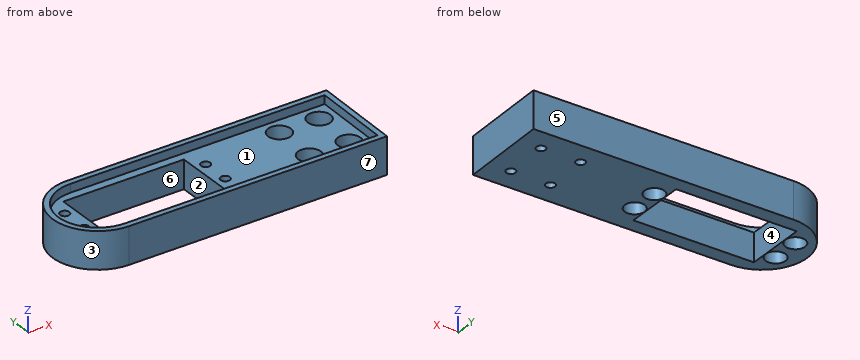
Autodesk Inventor part; units mm, degrees
ref_plane "YZ Plane" through (0, 0, 0) normal (1, 0, 0) x (0, 1, 0)
ref_plane "XZ Plane" through (0, 0, 0) normal (0, 1, 0) x (-1, 0, 0)
ref_plane "XY Plane" through (0, 0, 0) normal (0, 0, 1) x (1, 0, 0)
sketch "Szkic1" plane through (0, 0, 0) normal (0, 0, 1) x (1, 0, 0)
  line L0 (20.3, -9.9) -> (-20.3, -9.9)
  line L1 (-20.3, -9.9) -> (-20.3, 9.9)
  line L2 (-20.3, 9.9) -> (20.3, 9.9)
  line L3 (20.3, 9.9) -> (20.3, -9.9)
  line L4 (20.3, -9.9) -> (-20.3, 9.9) construction
  line L5 (-20.3, -9.9) -> (20.3, 9.9) construction
  line L6 (21.3, 10.9) -> (-21.3, 10.9)
  line L7 (-21.3, 10.9) -> (-21.3, -10.9)
  line L8 (-21.3, -10.9) -> (21.3, -10.9)
  line L9 (21.3, -10.9) -> (21.3, 10.9)
  line L10 (0, 0) -> (24.89, 0)
  line L11 (24.89, 0) -> (24.89, 5)
  line L12 (24.89, 5) -> (24.89, -5)
  line L13 (0, 0) -> (-24.89, 0)
  line L14 (-24.89, 5) -> (-24.89, 0)
  line L15 (-24.89, 0) -> (-24.89, -5)
  circle A0 centre (-24.89, 5) radius 1.621
  circle A1 centre (-24.89, -5) radius 1.621
  circle A2 centre (24.89, -5) radius 1.621
  circle A3 centre (24.89, 5) radius 1.621
  line L16 (-26.511, 5) -> (-31.511, 5)
  line L17 (26.511, 5) -> (31.511, 5)
  line L18 (0, 10.9) -> (0, 15.9)
  line L19 (0, 15.9) -> (-16.6819, 15.9)
  line L20 (0, -10.9) -> (0, -15.9)
  line L21 (0, -15.9) -> (-16.6819, -15.9)
  line L22 (-31.511, -5.7364) -> (-31.511, 5.7364)
  line L23 (0, 15.9) -> (31.511, 15.9)
  line L24 (31.511, 15.9) -> (31.511, -15.9)
  line L25 (0, -15.9) -> (31.511, -15.9)
  circle A4 centre (-16.6819, 0) radius 15.9
  arc A5 (-32.5353, -15.867) -> (-31.511, -15.9) centre (-31.511, 0) ccw
  line L26 (31.511, -15.9) -> (74.4699, -15.9)
  line L27 (74.4699, -15.9) -> (75.153, 15.9)
  line L28 (75.153, 15.9) -> (31.511, 15.9)
  point P0 (15.7555, -15.9)
  point P1 (29.1703, -29.1056)
  dimension "d10" = 3.242
  dimension "d13" = 3.242
  dimension "d0" = 40.6
  dimension "d1" = 19.8
  dimension "d2" = 1
  dimension "d3" = 42.6
  dimension "d4" = 24.89
  dimension "d5" = 5
  dimension "d6" = 10
  dimension "d7" = 24.89
  dimension "d8" = 5
  dimension "d9" = 5
  dimension "d11" = 3.242
  dimension "d12" = 3.242
  dimension "d14" = 5
  dimension "d15" = 5
  dimension "d16" = 5
  dimension "d17" = 5
  dimension "d18" = 6.621
  dimension "d19" = 63.022
  dimension "d20" = 10.9
  dimension "d21" = 0
extrude "Wyciągnięcie proste1" add sketch "Szkic1" along normal blind 10 contours A4 L22 L16 A0 L14 L13 L7 L8 | L8 L20 L21 A4 | L10 L11 A3 L17 L24 L25 L20 L8 L9 | L9 L6 L18 L23 L24 L17 A3 L11 L10 | L13 L14 A0 L16 L22 A4 L6 L7 | A4 L22 | A4 L19 L18 L6 | L24 L28 L27 L26
sketch "Szkic16" plane through (0, 0, 10) normal (0, 0, 1) x (1, 0, 0)
  line L0 (75.153, 15.9) -> (-16.6819, 15.9)
  arc A0 (-16.6819, 15.9) -> (-16.6819, -15.9) centre (-16.6819, 0) ccw
  line L1 (-16.6819, -15.9) -> (74.4699, -15.9)
  line L2 (74.4699, -15.9) -> (75.153, 15.9)
  circle A1 centre (24.89, 5) radius 1.621
  circle A2 centre (24.89, -5) radius 1.621
  line L3 (21.3, 10.9) -> (21.3, -10.9)
  line L4 (21.3, -10.9) -> (-21.3, -10.9)
  line L5 (-21.3, -10.9) -> (-21.3, 10.9)
  line L6 (-21.3, 10.9) -> (21.3, 10.9)
  circle A3 centre (-24.89, -5) radius 1.621
  circle A4 centre (-24.89, 5) radius 1.621
  line L7 (-16.6819, 13.9) -> (73.1096, 13.9)
  line L8 (73.1096, 13.9) -> (72.5124, -13.9)
  line L9 (72.5124, -13.9) -> (-16.6819, -13.9)
  arc A5 (-16.6819, 13.9) -> (-16.6819, -13.9) centre (-16.6819, 0) ccw
  point P0 (0, 0)
  dimension "d89" = 2
extrude "Wyciągnięcie proste9" add sketch "Szkic16" along normal blind 3 contours L2 L1 A0 L0
sketch "Szkic18" plane through (0, 0, 0) normal (0, 0, -1) x (-1, 0, 0)
  line L0 (-75.153, 15.9) -> (16.6819, 15.9)
  line L1 (16.6819, -15.9) -> (-74.4699, -15.9)
  line L2 (-74.4699, -15.9) -> (-75.153, 15.9)
  point P0 (0, 0)
  point P1 (-66.9793, 7.9)
  point P2 (-66.6399, -7.9)
  point P3 (-52.9793, 7.9)
  point P4 (-52.6399, -7.9)
  dimension "d94" = 8
  dimension "d95" = 8
  dimension "d105" = 8
  dimension "d106" = 8
  dimension "d107" = 14
  dimension "d108" = 14
  dimension "d109" = 8
  dimension "d110" = 8
hole "Otwór3" at (66.9793, 7.9, 0) at (66.6399, -7.9, 0) at (52.9793, 7.9, 0) at (52.6399, -7.9, 0) direction (0, 0, 1) diameter 3.242 end through all
sketch "Szkic19" plane through (0, 0, 10) normal (0, 0, 1) x (1, 0, 0)
  circle A0 centre (52.9793, 7.9) radius 1.621
  circle A1 centre (66.9793, 7.9) radius 1.621
  circle A2 centre (52.6399, -7.9) radius 1.621
  circle A3 centre (52.9793, 7.9) radius 1.621
  circle A4 centre (66.6399, -7.9) radius 1.621
  circle A5 centre (66.9793, 7.9) radius 1.621
  arc A6 (-16.6819, 13.9) -> (-16.6819, -13.9) centre (-16.6819, 0) ccw
  line L0 (-16.6819, -13.9) -> (72.5124, -13.9)
  line L1 (72.5124, -13.9) -> (73.1096, 13.9)
  line L2 (73.1096, 13.9) -> (-16.6819, 13.9)
  circle A7 centre (24.89, 5) radius 1.621
  circle A8 centre (24.89, -5) radius 1.621
  line L3 (21.3, 10.9) -> (21.3, -10.9)
  line L4 (21.3, -10.9) -> (-21.3, -10.9)
  line L5 (-21.3, -10.9) -> (-21.3, 10.9)
  line L6 (-21.3, 10.9) -> (21.3, 10.9)
  circle A9 centre (-24.89, -5) radius 1.621
  circle A10 centre (-24.89, 5) radius 1.621
  circle A11 centre (52.9793, 7.9) radius 4
  circle A12 centre (52.6399, -7.9) radius 4
  circle A13 centre (66.6399, -7.9) radius 4
  circle A14 centre (66.9793, 7.9) radius 4
  point P0 (0, 0)
  dimension "d111" = 8
  dimension "d112" = 8
  dimension "d113" = 8
  dimension "d114" = 8
extrude "Wyciągnięcie proste10" cut sketch "Szkic19" against normal blind 6 contours A2 | A11 | A12 | A13 | A14
sketch "Szkic20" plane through (0, 0, 0) normal (0, 0, -1) x (-1, 0, 0)
  circle A0 centre (-52.6399, -7.9) radius 1.621
  circle A1 centre (-52.9793, 7.9) radius 1.621
  circle A2 centre (-66.6399, -7.9) radius 1.621
  circle A3 centre (-66.9793, 7.9) radius 1.621
  line L0 (-75.153, 15.9) -> (16.6819, 15.9)
  line L1 (-74.4699, -15.9) -> (-75.153, 15.9)
  line L2 (16.6819, -15.9) -> (-74.4699, -15.9)
  arc A4 (16.6819, -15.9) -> (16.6819, 15.9) centre (16.6819, 0) ccw
  circle A5 centre (-24.89, 5) radius 1.621
  circle A6 centre (-24.89, -5) radius 1.621
  line L3 (-21.3, 10.9) -> (-21.3, -10.9)
  line L4 (21.3, 10.9) -> (-21.3, 10.9)
  line L5 (21.3, -10.9) -> (21.3, 10.9)
  line L6 (-21.3, -10.9) -> (21.3, -10.9)
  circle A7 centre (24.89, -5) radius 1.621
  circle A8 centre (24.89, 5) radius 1.621
  circle A9 centre (24.89, -5) radius 3.5
  circle A10 centre (24.89, 5) radius 3.5
  circle A11 centre (-24.89, -5) radius 3.5
  circle A12 centre (-24.89, 5) radius 3.5
  point P0 (0, 0)
  dimension "d117" = 7
  dimension "d118" = 7
  dimension "d119" = 7
  dimension "d120" = 7
extrude "Wyciągnięcie proste11" cut sketch "Szkic20" against normal blind 6 contours A5 | A6 | A7 | A8 | A9 | A10 | A11 | A12
equation "\"d13\" = d10"
equation "\"d11\" = d10"
equation "\"d12\" = d10"
properties part number "Ramie3_Drukowanie 3D"
Read the model definition and answer for the solid it produces. Units are mm, in the model's axes. Face numbers are marked on the shaded views. A direction names the side the tool comes from. Round coordinates to 2 decimals unless told otherwise and drop trailing zeros. Write each loop counter-clockwise with the first axis right and the second up, starting at its lowest first coordinate (ties: lowest second). Pieces come first, ordered by that corner, then holes. Notation, with made-up numbers: M 80,67.25 L 127,67.25 A23 ccw 127,93.25 Z; hole C 44.25,-29.5 d6. An arc over 180 degrees is marked long. Use a Markdown table: item, result.
1) Flat-ended cylindrical pins translate along their axes: pin 1 (9 mm diameter, centred on x = 66.98, y = 7.9, fed in from +Z); pin 2 (1 mm diameter, centred on y = 7.5, z = 3, fed in from +X); pin 3 (3 mm diameter, centred on x = 52.98, y = 7.9, fed in from +Z); pin 4 (7 mm diameter, centred on x = 52.98, y = 7.9, fed in from +Z). Find the tip coordinate at first contact, or state that the pin passes through.
Answers follow:
| item | result |
|---|---|
| pin 1 | stops at z = 10 |
| pin 2 | stops at x = 74.98 |
| pin 3 | passes through |
| pin 4 | stops at z = 4 |
2) The part is cut by section A-A (x = 61.5). Write down the section's boundary in (y, z).
Answers follow:
| item | result |
|---|---|
| outline | M -15.9,0 L 15.9,0 L 15.9,13 L 13.9,13 L 13.9,10 L -13.9,10 L -13.9,13 L -15.9,13 Z |
3) Straight lines are drawn through the part: line 1 along Y through (x, z) = (25, 7); line 2 along Y through (x, z) = (-5, 4); line 3 along Y through (x, z) = (-17, 11.75). For each, find the intervals that lie inside material, in ascending order. Write a range as [from, to].
Answers follow:
| item | result |
|---|---|
| line 1 | y = [-15.9, -6.62], [-3.38, 3.38], [6.62, 15.9] |
| line 2 | y = [-15.9, -10.9], [10.9, 15.9] |
| line 3 | y = [-15.9, -13.9], [13.9, 15.9] |
4) The part is cut by section B-B (z = 11.75). Write down the section's boundary in (x, y).
Answers follow:
| item | result |
|---|---|
| outline | M -16.68,-15.9 L 74.47,-15.9 L 75.15,15.9 L -16.68,15.9 A15.9 ccw Z; hole M -16.68,-13.9 L 72.51,-13.9 L 73.11,13.9 L -16.68,13.9 A13.9 ccw Z |
5) For a pull along Y with two mould halves and no side action, classify the marked faces 4, 5, 6 and 7 as pulls with the +Y half, pulls with the -Y half, needs draft (parallel to the pull), parting line crosses it, or undercut.
Answers follow:
| item | result |
|---|---|
| face 4 | undercut |
| face 5 | pulls with the +Y half |
| face 6 | undercut |
| face 7 | pulls with the -Y half |
6) The part is cut by section C-C (y = 0). Write down the section's boundary in (x, z).
Answers follow:
| item | result |
|---|---|
| outline | M -32.58,0 L -21.3,0 L -21.3,10 L -30.58,10 L -30.58,13 L -32.58,13 Z; M 21.3,0 L 74.81,0 L 74.81,13 L 72.81,13 L 72.81,10 L 21.3,10 Z |
7) A tool of negligible diameter and unlimited length cuts with its end or side. For the marked faces 1, 2 and 3, from which of +Z, -Z, +X, -X, +Y, -Y can it reach the whole face along a straight path? Write none if from no direction.
Answers follow:
| item | result |
|---|---|
| face 1 | +Z |
| face 2 | +Z, -Z |
| face 3 | +Z, -Z, -X |
8) The part is cut by section D-D (x = 4). Write down the section's boundary in (y, z).
Answers follow:
| item | result |
|---|---|
| outline | M -15.9,0 L -10.9,0 L -10.9,10 L -13.9,10 L -13.9,13 L -15.9,13 Z; M 10.9,0 L 15.9,0 L 15.9,13 L 13.9,13 L 13.9,10 L 10.9,10 Z |
